Verification items for the finished model (mm, model axes). A direction names the side the tool comes from. Coordinates: 2 decimals unless noted, no trailing zeros. Order: outer loops, then holes, each group sorted by start corner. A loop starts at its lowest first (then second) coordinate and runs counter-clockwise, first axis right, second up. Notation, with made-up numbers: M 57.25,87 L 82.25,87 A27 cw 82.25,120 Z; hole C 69,6.25 d4. An arc over 180 degrees is marked long. Return JSON: item names as keys, results as strings. Group by question number.
Q1. Section check C-C, the plane x = 5.65. Count the separate pieces of the cut face and the enclosed holes in it, then the cut area to 3 significant figures.
Q2. Section check A-A, the plane y = -107. Enter the section's corners in (x, z), then the cut area to 3 significant figures.
Q3. Access from +Z, -Z, +X, -X, +Y, -Y to the whole of each face (thin tool, end or side, straight path). Record for faces 1 (the face through (6.028, -146.524, 144.173)), 2 (the face through (8, -120, 87)).
Q4. Thickness scan on probe 1 along Z at (x, y) = (6.35, -158); probe 2 along Z at (x, y) = (6.35, -58); probe 3 along Y at (x, z) = (6.15, 31). Record the ranges inside material, lowest first.
Q5. Section check D-D, the plane y = -70. Enter the section's corners in (x, z), then the cut area to 3 significant figures.
Q6. Mould release check, pull along Z, two halves, no side actions. Record for faces 3 (the face through (6, -134, 10.496)), 4 (the face through (6.028, -57.759, 28.534)), 5 (the face through (6, -187.189, 150)): pulls with the +Z half, pulls with the -Z half, needs draft (parallel to the pull), parting line crosses it, or undercut.
Q7. Go/stop test with flat-tipped pins: pin 1 Ø2 at (x, y) = (6.5, -188.5) entering from -Z; pin 2 Ø1.5 at (y, z) = (-127.19, 153.73) entering from -X; pin 3 Ø2 at (x, z) = (5.5, 46.5) entering from +Y; pin 4 Ø1.5 at (x, y) = (7, -102.5) entering from +Z. Record where each tip stops, or that it passes through.
Q8. Section check B-B, the plane y = -159.5. Enter the section's corners in (x, z).
from build123d import *

# Parameters (mm, degrees)
AUFSATZ_LINEAR_AUSTRAGEN3_DEPTH      = 4
SCHNITT_LINEAR_AUSTRAGEN5_DEPTH      = 9.5
SCHNITT_LINEAR_AUSTRAGEN5_DEPTH_BACK = 9.5
SKIZZE2_24_R                         = 27
DURCHGANGSLOCH_F_R_M31_D             = 3.4
DURCHGANGSLOCH_F_R_M31_DEPTH         = 20
DURCHGANGSLOCH_F_R_M31_TIP           = 1.021463052
M3_GEWINDEBOHRUNG1_D                 = 2.5
M3_GEWINDEBOHRUNG1_DEPTH             = 8.5
M3_GEWINDEBOHRUNG1_TIP               = 0.751075774
SCHNITT_LINEAR_AUSTRAGEN6_DEPTH      = 11.5
SCHNITT_LINEAR_AUSTRAGEN7_DEPTH      = 251.552631004
SKIZZE13_W                           = 4
SKIZZE13_H                           = 30
AUFSATZ_LINEAR_AUSTRAGEN4_DEPTH      = 4


with BuildPart() as part:
    # Skizze2 → Aufsatz-Linear austragen3 (new body)
    with BuildSketch(Plane(origin=(0, 0, 0), x_dir=(0, 0, -1), z_dir=(1, 0, 0))):
        with BuildLine():
            Line((-10.496092502, -82.188867417), (-10.496092502, -187.188867417))
            Line((-10.496092502, -187.188867417), (-166.496092502, -187.188867417))
            Line((-166.496092502, -187.188867417), (-149.76794454, -72.118588605))
            ThreePointArc((-149.76794454, -72.118588605), (-75.447807774, -12.371141721), (-10.496092502, -82.188867417))
        make_face()
    extrude(amount=AUFSATZ_LINEAR_AUSTRAGEN3_DEPTH)

    # Skizze2<24> → Schnitt-Linear austragen5 (cut, two sides: drawn at the far end of the back side and taken through both)
    with BuildSketch(Plane(origin=(0, 0, 0), x_dir=(0, 0, -1), z_dir=(1, 0, 0)).offset(-SCHNITT_LINEAR_AUSTRAGEN5_DEPTH_BACK)):
        with Locations((-80.496092502, -82.188867417)):
            Circle(SKIZZE2_24_R)
    extrude(amount=SCHNITT_LINEAR_AUSTRAGEN5_DEPTH + SCHNITT_LINEAR_AUSTRAGEN5_DEPTH_BACK, mode=Mode.SUBTRACT)

    # Durchgangsloch für M31
    with Locations(Plane.ZY):
        with Locations((47.996092502, -82.188867417), (80.496092502, -49.688867417), (112.996092502, -82.188867417), (80.496092502, -114.688867417)):
            Hole(DURCHGANGSLOCH_F_R_M31_D / 2, depth=DURCHGANGSLOCH_F_R_M31_DEPTH)
            with Locations((0, 0, -(DURCHGANGSLOCH_F_R_M31_DEPTH + DURCHGANGSLOCH_F_R_M31_TIP / 2))):  # 118° drill point
                Cone(0, DURCHGANGSLOCH_F_R_M31_D / 2, DURCHGANGSLOCH_F_R_M31_TIP, mode=Mode.SUBTRACT)

    # M3 Gewindebohrung1
    with Locations(Plane.ZY):
        with Locations((33.827044944, -35.519819858), (103.069421962, -20.169154445), (14.496092502, -127.188867417), (14.496092502, -177.188867417), (147.189848539, -82.188867417), (153.731647743, -127.188867417)):
            Hole(M3_GEWINDEBOHRUNG1_D / 2, depth=M3_GEWINDEBOHRUNG1_DEPTH)
            with Locations((0, 0, -(M3_GEWINDEBOHRUNG1_DEPTH + M3_GEWINDEBOHRUNG1_TIP / 2))):  # 118° drill point
                Cone(0, M3_GEWINDEBOHRUNG1_D / 2, M3_GEWINDEBOHRUNG1_TIP, mode=Mode.SUBTRACT)

    # Skizze2<28> → Schnitt-Linear austragen6 (cut)
    with BuildSketch(Plane(origin=(0, 0, 0), x_dir=(0, 0, -1), z_dir=(1, 0, 0))):
        with BuildLine():
            Line((-25.496092502, -172.188916155), (-55.496092502, -172.188916155))
            ThreePointArc((-55.496092502, -172.188916155), (-62.567160314, -169.259983967), (-65.496092502, -162.188916155))
            Line((-65.496092502, -162.188916155), (-65.496092502, -146.461723273))
            Line((-65.496092502, -146.461723273), (-65.496092502, -136.73242799))
            ThreePointArc((-65.496092502, -136.73242799), (-63.912346618, -131.331810741), (-59.662759169, -127.641834561))
            ThreePointArc((-59.662759169, -127.641834561), (-54.057449416, -124.627035988), (-48.880535655, -120.924594661))
            ThreePointArc((-48.880535655, -120.924594661), (-45.913653233, -119.251775819), (-42.557424285, -118.67174011))
            Line((-42.557424285, -118.67174011), (-35.496092502, -118.67174011))
            ThreePointArc((-35.496092502, -118.67174011), (-28.425024691, -121.600672299), (-25.496092502, -128.67174011))
            Line((-25.496092502, -128.67174011), (-25.496092502, -172.188916155))
        make_face()
        with BuildLine():
            Line((-130.877768415, -111.399148996), (-125.911440332, -111.399148996))
            ThreePointArc((-125.911440332, -111.399148996), (-121.749137442, -112.3065567), (-118.342215694, -114.864102066))
            ThreePointArc((-118.342215694, -114.864102066), (-110.523367877, -122.168396348), (-101.329425836, -127.641834561))
            ThreePointArc((-101.329425836, -127.641834561), (-97.079838387, -131.331810741), (-95.496092502, -136.73242799))
            Line((-95.496092502, -136.73242799), (-95.496092502, -146.461723273))
            Line((-95.496092502, -146.461723273), (-95.496092502, -162.188916155))
            ThreePointArc((-95.496092502, -162.188916155), (-98.425024691, -169.259983967), (-105.496092502, -172.188916155))
            Line((-105.496092502, -172.188916155), (-135.495711073, -172.188916155))
            Line((-135.495711073, -172.188916155), (-147.455367056, -172.188916155))
            Line((-147.455367056, -172.188916155), (-140.79696332, -120.130459738))
            ThreePointArc((-140.79696332, -120.130459738), (-137.485079041, -113.892921828), (-130.877768415, -111.399148996))
        make_face()
    extrude(amount=SCHNITT_LINEAR_AUSTRAGEN6_DEPTH, mode=Mode.SUBTRACT)

    # Skizze12 → Schnitt-Linear austragen7 (cut, through all)
    with BuildSketch(Plane(origin=(0, 0, 0), x_dir=(0, -1, 0), z_dir=(-1, 0, 0))):
        with BuildLine():
            Line((31.912537744, 63.973777934), (30.971018966, 63.631093123))
            ThreePointArc((30.971018966, 63.631093123), (28.08654575, 60.904910522), (28.097068966, 56.936013123))
            ThreePointArc((28.097068966, 56.936013123), (38.550531474, 40.788465575), (53.642597032, 28.861700406))
            ThreePointArc((53.642597032, 28.861700406), (57.815417493, 28.555111356), (60.760235592, 31.52739563))
            Line((60.760235592, 31.52739563), (61.10653899, 32.478856395))
            ThreePointArc((61.10653899, 32.478856395), (61.093057729, 35.935652601), (58.840226031, 38.55755479))
            ThreePointArc((58.840226031, 38.55755479), (46.6574065, 48.223576562), (38.204358174, 61.277274988))
            ThreePointArc((38.204358174, 61.277274988), (35.592240185, 63.871037738), (31.912537744, 63.973777934))
        make_face()
        with BuildLine():
            Line((29.286912013, 88.138295897), (27.761021392, 88.693674664))
            ThreePointArc((27.761021392, 88.693674664), (25.233242691, 90.879922217), (24.8009776, 94.193906286))
            ThreePointArc((24.8009776, 94.193906286), (35.221155466, 116.203711215), (53.642597032, 132.130484599))
            ThreePointArc((53.642597032, 132.130484599), (57.815417493, 132.437073649), (60.760235592, 129.464789375))
            Line((60.760235592, 129.464789375), (61.10653899, 128.51332861))
            ThreePointArc((61.10653899, 128.51332861), (61.093057729, 125.056532404), (58.840226031, 122.434630215))
            ThreePointArc((58.840226031, 122.434630215), (43.883689457, 109.422090178), (35.461380891, 91.475254721))
            ThreePointArc((35.461380891, 91.475254721), (33.123794278, 88.419680828), (29.286912013, 88.138295897))
        make_face()
    extrude(amount=-SCHNITT_LINEAR_AUSTRAGEN7_DEPTH, mode=Mode.SUBTRACT)


with BuildPart() as body_2:
    # Spiegeln1: mirrored copy
    add(part.part.mirror(Plane(origin=(4, -82.188867417, 80.496092502), x_dir=(0, 0, 1), z_dir=(1, 0, 0))))

    # Skizze13 → Aufsatz-Linear austragen4 (add)
    with BuildSketch(Plane.XZ.offset(187.188867417)):
        with Locations((6, 57.496092502)):
            Rectangle(SKIZZE13_W, SKIZZE13_H)
        with Locations((6, 119.496092502)):
            Rectangle(SKIZZE13_W, SKIZZE13_H)
    extrude(amount=AUFSATZ_LINEAR_AUSTRAGEN4_DEPTH)


solid = body_2.part
Numbers:
{
 "1": {"separate pieces": "1", "enclosed holes": "15", "area": "15,600 mm2"},
 "2": {"outline": "M 4,10.5 L 8,10.5 L 8,69.85 L 4,69.85 Z; M 4,91.15 L 8,91.15 L 8,154.84 L 4,154.84 Z", "area": "492 mm2"},
 "3": {"face 1": "+X, -X", "face 2": "+Z, -Z, +X, +Y, -Y"},
 "4": {"probe 1": "z = 10.5 to 25.5, 65.5 to 95.5, 145.64 to 162.25", "probe 2": "z = 14.81 to 28.63, 39.04 to 68.5, 92.49 to 121.96, 132.36 to 146.18", "probe 3": "y = -187.19 to -172.19, -119.74 to -60.53, -50.08 to -32.69"},
 "5": {"outline": "M 4,11.57 L 8,11.57 L 8,56.4 L 4,56.4 Z; M 4,104.59 L 8,104.59 L 8,149.43 L 4,149.43 Z", "area": "359 mm2"},
 "6": {"face 3": "pulls with the -Z half", "face 4": "undercut", "face 5": "needs draft"},
 "7": {"pin 1": "stops at z = 42.5", "pin 2": "passes through", "pin 3": "stops at y = -20.45", "pin 4": "stops at z = 154.29"},
 "8": {"outline": "M 4,10.5 L 8,10.5 L 8,25.5 L 4,25.5 Z; M 4,65.5 L 8,65.5 L 8,95.5 L 4,95.5 Z; M 4,145.83 L 8,145.83 L 8,162.47 L 4,162.47 Z"}
}
